Here's how the part is built. I have some questions about the finished solid (model axes, mm). A direction names the side the tool comes from. Coordinates: 2 decimals unless noted, no trailing zeros. Loops run counter-clockwise (first coordinate to the right, second up) from the corner with the lowest first, then second, coordinate; pieces in that order, holes last. Notation, with made-up numbers: (72.25, 78) -> (122.25, 78) arc R21 cw to (122.25, 102) -> close; hole circle Ø1 at (81, -25.75). An arc over 180 degrees is marked (long way). Answer as a JSON object with one key per item and string values. Group by question number.
Q1. I want a section at A-A on z = 2. Count the separate pieces of the cut face and the enclosed holes in it, then the cut area to 3 significant figures.
Q2. I need wall thicknesses on line 1 (Y direction, x = 0, z = -2); line 2 (Z direction, x = -5.5, y = 53); line 3 (Y direction, x = -3.5, z = -8.5). Which ranges of each line are inside material? Lowest first, please.
Q3. I want a section at D-D on x = 0. Write out the boundary of the cut face in (y, z), then the cut area to 3 significant figures.
Q4. I want a section at C-C on x = 4. Write out the boundary of the cut face in (y, z), then the cut area to 3 significant figures.
Q5. On a 3-axis mill with a long thin cutter (end or side, diameter ignored), from which of +Z, -Z, +X, -X, +Y, -Y can I reach the whole of each face in a straight line? I mean faces 5 (the flat face through (2, 46, 0)), 6 (the cylindrical face through (-1.1, 48.7, -0.1)), 7 (the flat face through (-1, 55, -5)). Say none if no direction works.
Q6. I'm going to push flat-ended pins straight in: pin 1 (12 mm diameter, centred on y = 22, z = 1.5, fed in from -X); pin 2 (1.9 mm diameter, centred on y = 53, z = 0, fed in from -X); pin 3 (2 mm diameter, centred on x = -0.5, z = 2.5, fed in from +Y). Where does each tip first touch, or does it pass through?
Q7. I want a section at B-B on y = 23. Write out the boundary of the cut face in (x, z), then the cut area to 3 significant figures.
Q8. Thinking about a two-plate mould opening in Z: for faces 1 (the flat face through (9, 1, 0)), 2 (the cylindrical face through (-0.14, 18.3, 2.45)), 3 (the flat face through (9, 27, 9)), 4 (the flat face through (9, 27, -9)), which applies, released by +Z, released by -Z, zero draft, split by the parting line, or undercut?
```python
from build123d import *

# Parameters (mm, degrees)
SKETCH1_W               = 20
SKETCH1_H               = 20
BOSS_EXTRUDE1_DEPTH     = 55
CUT_EXTRUDE1_DEPTH      = 60.371710435
CUT_EXTRUDE1_DEPTH_BACK = 60.371710435
SKETCH2_R               = 5.3
SKETCH2_W               = 4
SKETCH2_H               = 3
SKETCH3_R               = 5.3
CUT_EXTRUDE2_DEPTH      = 60.371710435
SKETCH4_R               = 4.3
CUT_EXTRUDE3_DEPTH      = 18
CHAMFER1_SIZE           = 2


with BuildPart() as part:
    # Sketch1 → Boss-Extrude1 (new body)
    with BuildSketch(Plane(origin=(0, 0, 0), x_dir=(1, 0, 0), z_dir=(0, 1, 0))):
        Rectangle(SKETCH1_W, SKETCH1_H)
    extrude(amount=BOSS_EXTRUDE1_DEPTH)

    # Sketch2 → Cut-Extrude1 (cut, two sides: drawn at the far end of the back side and taken through both)
    with BuildSketch(Plane.XY.offset(10).offset(-CUT_EXTRUDE1_DEPTH_BACK)):
        with Locations((0, 12)):
            Circle(SKETCH2_R)
        with Locations((0, 34)):
            Circle(SKETCH2_R)
        with Locations((0, 46.5)):
            Rectangle(SKETCH2_W, SKETCH2_H)
    extrude(amount=CUT_EXTRUDE1_DEPTH + CUT_EXTRUDE1_DEPTH_BACK, mode=Mode.SUBTRACT)

    # Sketch3 → Cut-Extrude2 (cut, through all)
    with BuildSketch(Plane.ZY.offset(10)):
        with Locations((0, 23)):
            Circle(SKETCH3_R)
    extrude(amount=-CUT_EXTRUDE2_DEPTH, mode=Mode.SUBTRACT)

    # Sketch4 → Cut-Extrude3 (cut)
    with BuildSketch(Plane.ZY.offset(10)):
        with Locations((0, 53)):
            Circle(SKETCH4_R)
    extrude(amount=-CUT_EXTRUDE3_DEPTH, mode=Mode.SUBTRACT)

    # Chamfer1
    chamfer1_edges = [part.edges().sort_by_distance(p)[0] for p in [
        (10, 55, 0),
        (0, 55, -10),
        (0, 0, -10),
        (10, 0, 0),
        (0, 0, 10),
        (0, 55, 10),
        (10, 27.5, -10),
        (10, 27.5, 10),
    ]]
    chamfer(chamfer1_edges, length=CHAMFER1_SIZE - 0.0001)  # a hair under: the kernel refuses the full size


solid = part.part
```
Result set:
{
 "1": {"separate pieces": "2", "enclosed holes": "3", "area": "607 mm²"},
 "2": {"line 1": "y = 0 to 6.7, 17.3 to 18.09, 27.91 to 28.7, 39.3 to 45, 48 to 49.19", "line 2": "z = -10 to -4.3, 4.3 to 10", "line 3": "y = 0.5 to 8.02, 15.98 to 30.02, 37.98 to 54.5"},
 "3": {"outline": "(0, -8) -> (2, -10) -> (6.7, -10) -> (6.7, 10) -> (2, 10) -> (0, 8) -> close; (17.3, -10) -> (28.7, -10) -> (28.7, 10) -> (17.3, 10) -> close; (39.3, -10) -> (45, -10) -> (45, 10) -> (39.3, 10) -> close; (48, -10) -> (53, -10) -> (55, -8) -> (55, -3.81) arc R4.3 cw (long way) to (55, 3.81) -> (55, 8) -> (53, 10) -> (48, 10) -> close; hole circle Ø10.6 at (23, 0)", "area": "474 mm²"},
 "4": {"outline": "(0, -8) -> (2, -10) -> (8.52, -10) -> (8.52, 10) -> (2, 10) -> (0, 8) -> close; (15.48, -10) -> (30.52, -10) -> (30.52, 10) -> (15.48, 10) -> close; (37.48, -10) -> (53, -10) -> (55, -8) -> (55, -3.81) arc R4.3 cw (long way) to (55, 3.81) -> (55, 8) -> (53, 10) -> (37.48, 10) -> close; hole circle Ø10.6 at (23, 0)", "area": "680 mm²"},
 "5": {"face 5": "+Z, -Z", "face 6": "-X", "face 7": "+Z, -Z, +X, -X, +Y"},
 "6": {"pin 1": "stops at x = -10", "pin 2": "stops at x = 8", "pin 3": "stops at y = 50.5"},
 "7": {"outline": "(-10, -10) -> (8, -10) -> (10, -8) -> (10, -5.3) -> (-10, -5.3) -> close; (-10, 5.3) -> (10, 5.3) -> (10, 8) -> (8, 10) -> (-10, 10) -> close", "area": "184 mm²"},
 "8": {"face 1": "zero draft", "face 2": "undercut", "face 3": "released by +Z", "face 4": "released by -Z"}
}
